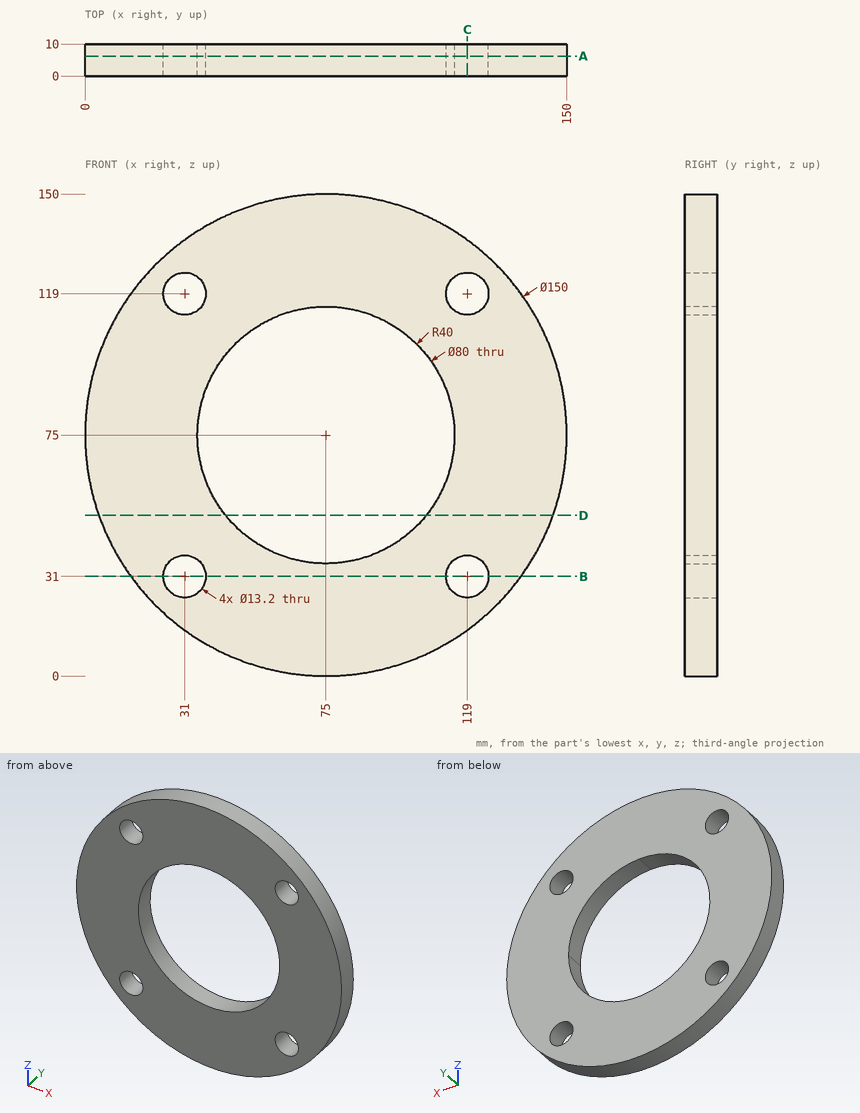
Part print with two shaded views. Sizes in mm from the minimum x, y, z corner. Coordinates: 2 decimals unless noted, no trailing zeros. Write each loop counter-clockwise with the first axis right and the second up, starting at its lowest first coordinate (ties: lowest second). Pieces come first, ordered by that corner, then holes. Notation, with made-up numbers: (79.5, 13) - (137.5, 13) arc R23 ccw to (137.5, 26) - close; hole circle Ø11 at (-33.5, 0.25). An arc over 180 degrees is marked (long way). Use a Markdown table: item, result. Add a question column.
Item 1: Band-saw the part on C-C, the plane x = 119. Write the cut outline in (y, z).
Item 2: Drill centre lines: line 1 along X through (y, z) = (8.75, 118); line 2 along Z through (x, y) = (125, 9.25); line 3 along X through (y, z) = (4, 117). Where is each one in solid material? Low to high.
Item 3: Drop flat-ended pins along their axis: pin 1 (1 mm diameter, centred on y = 2.5, z = 15.5, fed in from +X); pin 2 (1 mm diameter, centred on y = 7.5, z = 104, fed in from +X); pin 3 (8 mm diameter, centred on x = 119, z = 119, fed in from +Y); pin 4 (4 mm diameter, centred on x = 25.5, y = 1.5, fed in from -Z). Give the stop position or say it passes through.
Item 4: Band-saw the part on A-A, the plane y = 6.25. Write the cut outline in (x, z).
Item 5: Band-saw the part on B-B, the plane z = 31. Write the cut outline in (x, y).
Item 6: Band-saw the part on D-D, the plane z = 50. Write the cut outline in (x, y).
A:
| question | item | result |
|---|---|---|
| 1 | outline | (0, 14.26) - (10, 14.26) - (10, 24.4) - (0, 24.4) - close; (0, 37.6) - (10, 37.6) - (10, 112.4) - (0, 112.4) - close; (0, 125.6) - (10, 125.6) - (10, 135.74) - (0, 135.74) - close |
| 2 | line 1 | x = 13.55 to 24.48, 37.52 to 112.48, 125.52 to 136.45 |
| 2 | line 2 | z = 19.1 to 28.25, 33.75 to 116.25, 121.75 to 130.9 |
| 2 | line 3 | x = 12.86 to 24.71, 37.29 to 112.71, 125.29 to 137.14 |
| 3 | pin 1 | stops at x = 121.3 |
| 3 | pin 2 | stops at x = 144.37 |
| 3 | pin 3 | passes through |
| 3 | pin 4 | stops at z = 16.96 |
| 4 | outline | circle Ø150 at (75, 75); hole circle Ø13.2 at (31, 31); hole circle Ø13.2 at (31, 119); hole circle Ø80 at (75, 75); hole circle Ø13.2 at (119, 31); hole circle Ø13.2 at (119, 119) |
| 5 | outline | (14.26, 0) - (24.4, 0) - (24.4, 10) - (14.26, 10) - close; (37.6, 0) - (112.4, 0) - (112.4, 10) - (37.6, 10) - close; (125.6, 0) - (135.74, 0) - (135.74, 10) - (125.6, 10) - close |
| 6 | outline | (4.29, 0) - (43.78, 0) - (43.78, 10) - (4.29, 10) - close; (106.22, 0) - (145.71, 0) - (145.71, 10) - (106.22, 10) - close |
